```python
from build123d import *

# Parameters (mm, degrees)
CROQUIS2_W              = 3
CROQUIS2_H              = 7
SALIENTE_EXTRUIR1_DEPTH = 3
CROQUIS3_W              = 7
CROQUIS3_H              = 3
CORTAR_EXTRUIR1_DEPTH   = 3
SALIENTE_EXTRUIR2_DEPTH = 3


with BuildPart() as part:
    # Croquis2 → Saliente-Extruir1 (new body)
    with BuildSketch(Plane.XY):
        with BuildLine():
            ThreePointArc((28.504213464, 6.97614846), (38.823203621, 10.80038439), (48, 16.874324342))
            Line((48, 16.874324342), (48, 18.374324342))
            Line((48, 18.374324342), (45, 18.374324342))
            Line((45, 18.374324342), (45, 22.874324342))
            Line((45, 22.874324342), (48, 22.874324342))
            Line((48, 22.874324342), (48, 27.374324342))
            Line((48, 27.374324342), (45.958765785, 27.374324342))
            ThreePointArc((45.958765785, 27.374324342), (32.608459646, 17.819059857), (16.508760518, 14.604492799))
            add(Edge.make_bspline(
                [(0, 23.003403927), (3.768895236, 21.748521109), (6.947387732, 20.10306336), (11.1476301, 16.408164217), (14.028002641, 14.311208734), (16.508760518, 14.604492799)],
                knots=[0, 0, 0, 0, 0.366175843, 0.466175843, 1, 1, 1, 1], degree=3))
            Line((0, 23.003403927), (0, 16.003403927))
            Line((0, 16.003403927), (0, 7))
            Line((0, 7), (0, 0))
            Line((0, 0), (28.504213464, 6.97614846))
        make_face()
        with Locations((-1.5, 3.5)):
            Rectangle(CROQUIS2_W, CROQUIS2_H)
        with Locations((-1.5, 19.503403927)):
            Rectangle(CROQUIS2_W, CROQUIS2_H)
    extrude(amount=SALIENTE_EXTRUIR1_DEPTH)

    # Croquis3 → Cortar-Extruir1 (cut)
    with BuildSketch(Plane.XY):
        with Locations((18.5, 8.5)):
            Rectangle(CROQUIS3_W, CROQUIS3_H)
    extrude(amount=CORTAR_EXTRUIR1_DEPTH, mode=Mode.SUBTRACT)

    # Croquis4 → Saliente-Extruir2 (add)
    with BuildSketch(Plane.XY):
        with BuildLine():
            Line((45, 18.374324342), (45, 14.546008954))
            ThreePointArc((45, 14.546008954), (44.879211841, 14.45997986), (44.758158478, 14.374324342))
            Line((44.758158478, 14.374324342), (48, 14.374324342))
            Line((48, 14.374324342), (48, 18.374324342))
            Line((48, 18.374324342), (45, 18.374324342))
        make_face()
    extrude(amount=SALIENTE_EXTRUIR2_DEPTH)


solid = part.part
```
Here's how the part is built. I have some questions about the finished solid (model axes, mm). A direction names the side the tool comes from. Give positions to 0.01 mm unless a question says otherwise; leave off trailing zeros. Loops run counter-clockwise (first coordinate to the right, second up) from the corner with the lowest first, then second, coordinate; pieces in that order, holes last. Notation, with made-up numbers: M 56.25,-13.75 L 77.25,-13.75 A9 cw 77.25,-1.75 Z; hole C 69,62 d2. An arc over 180 degrees is marked long. Put each result on its own line as item: value. Start each with the question number.
(1) I want a section at C-C on y = 25. Please give me the cut outline in (x, z), then the cut area to 3 significant figures.
(2) I need wall thicknesses on line 1 along Y through (x, z) = (17, 2.25); line 2 along X through (y, z) = (19.5, 2.5); line 3 along Y through (x, z) = (19, 2.5). Which ranges of each line are inside material? Lowest first, please. Write a range as [from, to].
(3) Will these pins go through, and if not, where does the flat tip stop? pin 1 Ø10 at (x, y) = (21, 21) entering from -Z; pin 2 Ø0.9 at (x, z) = (18.5, 1.5) entering from +Y; pin 3 Ø1.5 at (y, z) = (8.5, 2) entering from -X; pin 4 Ø1.5 at (x, z) = (42.5, 2.5) entering from -Y.
(4) If we mould it in two halves opening along X, with no side actions, what happens to faces 1 (the flat face through (-2, 0, 1)), 2 (the flat face through (48, 25, 1)), 3 (the flat face through (15, 8, 1)), 4 (the cylindrical face through (32.82, 17.91, 1.48))? For each: +X half, -X half, draft (parallel to the pull), parting line (faces both ways), or undercut.
(5) I want a section at D-D on x = 43. Please give me the cut outline in (y, z).
(6) I want a section at A-A on x = 18. Please give me the cut outline in (y, z), then the cut area to 3 significant figures.
(7) I want a section at B-B on y = 9.5. Please give me the cut outline in (x, z), then the cut area to 3 significant figures.
(8) For faces 5 (the flat face through (18, 10, 1)), 6 (the flat face through (0, 12, 1)), 7 (the flat face through (47, 18.374, 1)), which set-ups out of +Z, -Z, +X, -X, +Y, -Y let a thin tool reach every point of the face, with its end or its side?
Answer block:
1. outline: M 43.61,0 L 48,0 L 48,3 L 43.61,3 Z
1. area: 13.2 mm^2
2. line 1: [4.16, 7], [10, 14.6]
2. line 2: [-3, 7.49], [36.02, 45]
2. line 3: [4.65, 7], [10, 14.65]
3. pin 1: through
3. pin 2: y = 14.64
3. pin 3: x = 0
3. pin 4: y = 12.42
4. face 1: draft
4. face 2: +X half
4. face 3: undercut
4. face 4: undercut
5. outline: M 13.19,0 L 24.45,0 L 24.45,3 L 13.19,3 Z
6. outline: M 4.41,0 L 7,0 L 7,3 L 4.41,3 Z; M 10,0 L 14.61,0 L 14.61,3 L 10,3 Z
6. area: 21.6 mm^2
7. outline: M 0,0 L 15,0 L 15,3 L 0,3 Z; M 22,0 L 36.05,0 L 36.05,3 L 22,3 Z
7. area: 87.1 mm^2
8. face 5: +Z, -Z
8. face 6: +Z, -Z, -X
8. face 7: +Z, -Z, +X
